Design review of the part built by this model. Coordinates are the model's own, in mm. Face numbers are marked on the shaded views. Coordinates: 2 decimals unless noted, no trailing zeros. Loops run counter-clockwise (first coordinate to the right, second up) from the corner with the lowest first, then second, coordinate; pieces in that order, holes last. Notation, with made-up numbers: (-20, 10) -> (1, 10) arc R36 ccw to (1, 47) -> close; hole circle Ø8 at (-30.5, 36). An arc over 180 degrees is marked (long way). One line per item, written item: value. Start each with the question number.
1. Insertion check: pin 1 (1.5 mm diameter, centred on y = -8, z = 41, fed in from +X); pin 2 (1.5 mm diameter, centred on x = -2.5, z = 78, fed in from +Y); pin 3 (5 mm diameter, centred on y = -10, z = 87, fed in from -X). Each pin has a flat end and moves straight along its axis. Give the tip position at first contact, or say it passes through.
2. Draft analysis for pull direction Y (two halves, no side actions). For the marked faces 1 and 2, state which applies: pulls with the +Y half, pulls with the -Y half, needs draft (parallel to the pull), parting line crosses it, or undercut.
3. Add section A-A on x = 0. Write out the cut boundary in (y, z).
4. Add section B-B on y = -4.75. Write out the cut boundary in (x, z), plus the area to 3 significant figures.
5. Add section C-C on x = 10.5. Write out the cut boundary in (y, z).
6. For probe 1 along X at (y, z) = (6.5, 37); probe 2 along X at (y, z) = (-1, 12.5); probe 3 along Y at (x, z) = (-11, 18.5), list the stretches that pass through material, from the lowest coordinate up.
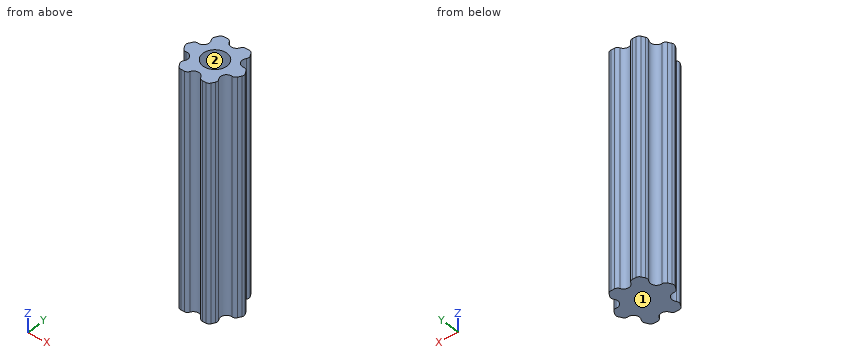
```python
from build123d import *

# Parameters (mm, degrees)
PAD_DEPTH       = 120
SKETCH001_R     = 6.1
POCKET_DEPTH    = 40
SKETCH002_R     = 3
POCKET001_DEPTH = 120.001
FILLET_R        = 2


with BuildPart() as part:
    # Sketch → Pad (new body)
    with BuildSketch(Plane.XY):
        Polygon((-7.5, -12.990381), (7.5, -12.990381), (15, 0), (7.5, 12.990381), (-7.5, 12.990381), (-15, 0), align=None)
    extrude(amount=PAD_DEPTH)

    # Sketch001 (on Face8 of Pad) → Pocket (cut)
    with BuildSketch(Plane.XY.offset(120)):
        Circle(SKETCH001_R)
    extrude(amount=-POCKET_DEPTH, mode=Mode.SUBTRACT)

    # Sketch002 (on Face5 of Pocket) → Pocket001 (cut, through all)
    with BuildSketch(Plane.XY.offset(120)):
        with Locations((-11.25, 6.495191)):
            Circle(SKETCH002_R)
        with Locations((0, 12.990381)):
            Circle(SKETCH002_R)
        with Locations((11.25, 6.495191)):
            Circle(SKETCH002_R)
        with Locations((11.25, -6.495191)):
            Circle(SKETCH002_R)
        with Locations((0, -12.990381)):
            Circle(SKETCH002_R)
        with Locations((-11.25, -6.495191)):
            Circle(SKETCH002_R)
    extrude(amount=-POCKET001_DEPTH, mode=Mode.SUBTRACT)

    # Fillet
    fillet_edges = [part.edges().sort_by_distance(p)[0] for p in [
        (-9.75, 9.093267, 60),
        (-3, 12.990381, 60),
        (-7.5, 12.990381, 60),
        (3, 12.990381, 60),
        (7.5, 12.990381, 60),
        (-15, 0, 60),
        (-12.75, 3.897114, 60),
        (-12.75, -3.897114, 60),
        (9.75, 9.093267, 60),
        (12.75, 3.897114, 60),
        (15, 0, 60),
        (12.75, -3.897114, 60),
        (9.75, -9.093267, 60),
        (7.5, -12.990381, 60),
        (3, -12.990381, 60),
        (-3, -12.990381, 60),
        (-7.5, -12.990381, 60),
        (-9.75, -9.093267, 60),
    ]]
    fillet(fillet_edges, radius=FILLET_R)


solid = part.part
```
Worked answers:
1. pin 1: stops at x = 9.09
1. pin 2: stops at y = 12.48
1. pin 3: stops at x = -9.23
2. face 1: needs draft
2. face 2: undercut
3. outline: (-9.99, 0) -> (9.99, 0) -> (9.99, 120) -> (6.1, 120) -> (6.1, 80) -> (-6.1, 80) -> (-6.1, 120) -> (-9.99, 120) -> close
4. outline: (-8.81, 0) -> (8.81, 0) -> (8.81, 120) -> (3.83, 120) -> (3.83, 80) -> (-3.83, 80) -> (-3.83, 120) -> (-8.81, 120) -> close
4. area: 1,810 mm²
5. outline: (-3.59, 0) -> (3.59, 0) -> (3.59, 120) -> (-3.59, 120) -> close
6. probe 1: x = -8.25 to 8.25
6. probe 2: x = -14.42 to 14.42
6. probe 3: y = -3.51 to 3.51
